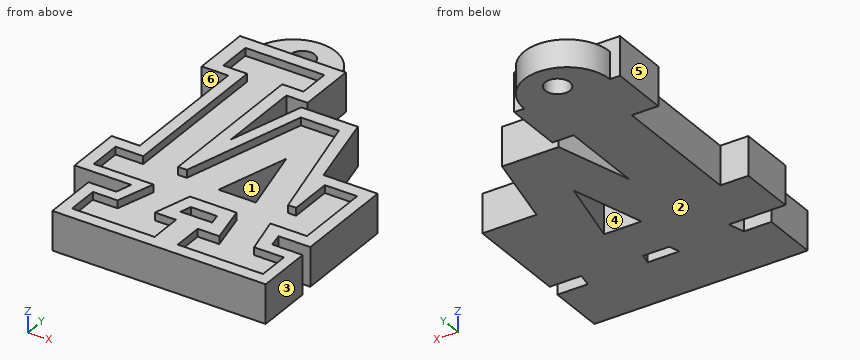
from build123d import *

# Parameters (mm, degrees)
F1_DEPTH = 5
F0_R     = 1.5875
F2_DEPTH = 3.5
F3_DEPTH = 4


with BuildPart() as f1:
    # F0 (on Top) → F1 (new body)
    with BuildSketch(Plane.XY):
        Polygon((-14.761455, 21.829162), (-16.066568, 21.829162), (-16.066568, 14.353847), (-12.664012, 14.353847), (-12.664012, -2.916705), (-16.272783, -2.916705), (-16.272783, -10.13425), (-9.003686, -10.13425), (-9.570778, -12.196405), (-13.127998, -12.196405), (-13.127998, -19.259289), (14.298672, -19.259289), (14.298672, -12.041744), (10.380576, -12.041744), (10.019699, -10.237358), (14.092457, -10.237358), (14.092457, 2.908884), (7.132681, 2.908884), (4.761202, 13.219662), (-2.507896, 13.219662), (-5.188699, 3.527531), (-5.188699, 14.353848), (-2.456342, 14.353848), (-2.456342, 21.829162), (-3.761455, 21.829162), align=None)
        Polygon((-1.53564, -11.828732), (-1.14685, -10.423108), (2.212943, -10.423108), (2.539253, -11.828732), align=None, mode=Mode.SUBTRACT)
        Polygon((-14.241549, 15.777845), (-14.241549, 20.112993), (-4.097303, 20.112993), (-4.097303, 16.037954), (-6.828447, 16.037954), (-6.828447, -4.293891), (-5.701307, -4.293891), (-1.409511, 11.442697), (3.489206, 11.442697), (7.347488, -4.337242), (8.387923, -4.337242), (8.387923, 1.255099), (12.549666, 1.255099), (12.549666, -8.542337), (7.824354, -8.542337), (9.081547, -13.571107), (12.896478, -13.571107), (12.896478, -17.646147), (1.928553, -17.646147), (1.928553, -13.744514), (4.703048, -13.744514), (3.575909, -8.672391), (-2.406595, -8.672391), (-3.750491, -13.484405), (-1.019347, -13.484405), (-1.019347, -17.689498), (-11.640461, -17.689498), (-11.640461, -13.61446), (-8.475802, -13.61446), (-7.045203, -8.759094), (-14.718415, -8.759094), (-14.718415, -4.510649), (-11.163594, -4.510649), (-11.163594, 15.777845), align=None, mode=Mode.SUBTRACT)
    extrude(amount=F1_DEPTH)

    # F0 (on Top) → F2 (join)
    with BuildSketch(Plane.XY):
        with BuildLine():
            ThreePointArc((-3.761455, 21.829162), (-9.261455, 27.329162), (-14.761455, 21.829162))
            Line((-14.761455, 21.829162), (-3.761455, 21.829162))
        make_face()
        with Locations((-9.261455, 23.674398)):
            Circle(F0_R, mode=Mode.SUBTRACT)
    extrude(amount=F2_DEPTH)

    # F0 (on Top) → F3 (join)
    with BuildSketch(Plane.XY):
        Polygon((-4.097303, 20.112993), (-14.241549, 20.112993), (-14.241549, 15.777845), (-11.163594, 15.777845), (-11.163594, -4.510649), (-14.718415, -4.510649), (-14.718415, -8.759094), (-7.045203, -8.759094), (-8.475802, -13.61446), (-11.640461, -13.61446), (-11.640461, -17.689498), (-1.019347, -17.689498), (-1.019347, -13.484405), (-3.750491, -13.484405), (-2.406595, -8.672391), (3.575909, -8.672391), (4.703048, -13.744514), (1.928553, -13.744514), (1.928553, -17.646147), (12.896478, -17.646147), (12.896478, -13.571107), (9.081547, -13.571107), (7.824354, -8.542337), (12.549666, -8.542337), (12.549666, 1.255099), (8.387923, 1.255099), (8.387923, -4.337242), (7.347488, -4.337242), (3.489206, 11.442697), (-1.409511, 11.442697), (-5.701307, -4.293891), (-6.828447, -4.293891), (-6.828447, 16.037954), (-4.097303, 16.037954), align=None)
        Polygon((-1.515705, -4.444579), (1.059277, 4.864968), (3.282977, -4.444579), align=None, mode=Mode.SUBTRACT)
    extrude(amount=F3_DEPTH)


solid = f1.part
Verification items for the finished model (mm, model axes). Face numbers are marked on the shaded views. A direction names the side the tool comes from. Give positions to 0.01 mm unless a question says otherwise; leave off trailing zeros. Loops run counter-clockwise (first coordinate to the right, second up) from the corner with the lowest first, then second, coordinate; pieces in that order, holes last.
1. Cross-section at D-D on z = 1.2. Count the separate pieces of the cut face and the enclosed holes in it, and give its area (3 significant figures).
Derived:
separate pieces: 1
enclosed holes: 3
area: 911 mm2
2. Cross-section at C-C on y = 6. Record the cut outline in (x, z), and give its area (3 significant figures).
Derived:
outline: (-12.66, 0) - (-5.19, 0) - (-5.19, 5) - (-6.83, 5) - (-6.83, 4) - (-11.16, 4) - (-11.16, 5) - (-12.66, 5) - close; (-4.5, 0) - (6.42, 0) - (6.42, 5) - (4.82, 5) - (4.82, 4) - (-2.89, 4) - (-2.89, 5) - (-4.5, 5) - close
area: 80.0 mm2
3. Tool access check on the marked faces 4, 5 and 6. Record the directions out of +Z, -Z, +X, -X, +Y, -Y that give a thin tool (end or side, any length) a straight path to the whole face; none if there is none.
Derived:
face 4: +Z, -Z
face 5: +Z, -Z, -X, +Y
face 6: +Z, -Z, -X
4. Go/stop test with flat-tipped pins: P1, Ø1.1, axis at x = -11.5, z = 1.5, coming from the +Y side; P2, Ø0.5, axis at y = -16, z = 4.5, coming from the -X side; P3, Ø1.1, axis at y = -1.5, z = 4.5, coming from the -X side; P4, Ø6, axis at x = 7, y = 18, coming from the -Z side. Record where each tip stops, or that it passes through.
Derived:
P1: stops at y = 27.06
P2: stops at x = -13.13
P3: stops at x = -12.66
P4: passes through
5. Cross-section at A-A on y = -16. Record the cut outline in (x, z).
Derived:
outline: (-13.13, 0) - (14.3, 0) - (14.3, 5) - (12.9, 5) - (12.9, 4) - (1.93, 4) - (1.93, 5) - (-1.02, 5) - (-1.02, 4) - (-11.64, 4) - (-11.64, 5) - (-13.13, 5) - close
6. Cross-section at B-B on x = 0. Record the cut outline in (y, z).
Derived:
outline: (-19.26, 0) - (-11.83, 0) - (-11.83, 5) - (-19.26, 5) - close; (-10.42, 0) - (-4.44, 0) - (-4.44, 4) - (-8.67, 4) - (-8.67, 5) - (-10.42, 5) - close; (1.04, 0) - (13.22, 0) - (13.22, 5) - (11.44, 5) - (11.44, 4) - (1.04, 4) - close
7. Material ranges on probe 1 along Y at (x, z) = (-14, 4.2); probe 2 along Y at (x, z) = (-15, 3.5); probe 3 along X at (y, z) = (13, 4.3), recorded low to high.
Derived:
probe 1: y = -10.13 to -8.76, -4.51 to -2.92, 14.35 to 15.78, 20.11 to 21.83
probe 2: y = -10.13 to -2.92, 14.35 to 21.83
probe 3: x = -12.66 to -11.16, -6.83 to -5.19, -2.57 to 4.81
8. Release check for a two-part mould opening along X. For the marked faces 1, 2 and 3 record: +X half, -X half, draft (parallel to the pull), parting line (faces both ways), or undercut.
Derived:
face 1: undercut
face 2: draft
face 3: +X half
